Autodesk Inventor part; units mm, degrees
ref_plane "YZ Plane" through (0, 0, 0) normal (1, 0, 0) x (0, 1, 0)
ref_plane "XZ Plane" through (0, 0, 0) normal (0, 1, 0) x (-1, 0, 0)
ref_plane "XY Plane" through (0, 0, 0) normal (0, 0, 1) x (1, 0, 0)
sketch "Эскиз1" plane through (0, 0, 0) normal (0, 0, 1) x (1, 0, 0)
  circle A0 centre (-3.8814, -5.2176) radius 1.5
  line L0 (-10.8201, 1.8432) -> (-11.0949, -29.6556)
  line L1 (4.4719, -79.3628) -> (5.5191, 40.6326)
  line L2 (-9.8587, -12.7657) -> (-5.4656, -12.804)
  line L3 (-10.9475, -12.7562) -> (5.315, -12.7562)
  line L4 (5.315, -12.7562) -> (5.315, 17.2438)
  line L5 (5.315, 17.2438) -> (-10.9475, 17.2438)
  line L6 (-10.9475, 17.2438) -> (-10.9475, -12.7562)
  point P0 (0, 0)
  point P1 (5.1784, 1.5986)
  point P2 (5.0531, -12.7562)
  dimension "d0" = 30
extrude "Выдавливание1" add sketch "Эскиз1" along normal blind 3 contours L3 L6 L5 L1
sketch "Эскиз2" plane through (5.315, 17.2438, 3) normal (1, -0.0087, 0) x (0, 0, -1)
  spline S0 degree 3 poles (-15.9024, -5.0587) (-16.7308, -5.0587) (-17.4024, -4.3871) (-17.4024, -3.5587) (-17.4024, -2.7303) (-16.7308, -2.0587) (-15.9024, -2.0587) (-15.074, -2.0587) (-14.4024, -2.7303) (-14.4024, -3.5587) (-14.4024, -4.3871) (-15.074, -5.0587) (-15.9024, -5.0587) knots 0 0 0 0 0.25 0.25 0.25 0.5 0.5 0.5 0.75 0.75 0.75 1 1 1 1
  spline S1 degree 3 poles (-20.7708, 4.5722) (-21.5992, 4.5722) (-22.2708, 5.2438) (-22.2708, 6.0722) (-22.2708, 6.9006) (-21.5992, 7.5722) (-20.7708, 7.5722) (-19.9424, 7.5722) (-19.2708, 6.9006) (-19.2708, 6.0722) (-19.2708, 5.2438) (-19.9424, 4.5722) (-20.7708, 4.5722) knots 0 0 0 0 0.25 0.25 0.25 0.5 0.5 0.5 0.75 0.75 0.75 1 1 1 1
  line L0 (0, -30.0011) -> (0, 0)
  line L1 (0, -7.2902) -> (-26.751, -7.2902)
  spline S2 degree 3 poles (-117.3896, -42.4533) (-114.4523, -72.8485) (-88.8364, -96.6103) (-57.6706, -96.6103) (-24.5335, -96.6103) (2.3293, -69.7475) (2.3293, -36.6104) (2.3293, -3.4733) (-24.5335, 23.3896) (-57.6706, 23.3896) (-89.3782, 23.3896) (-115.3412, -1.2057) (-117.5222, -32.3587) knots 0 0 0 0 0.2 0.2 0.2 0.4 0.4 0.4 0.6 0.6 0.6 0.8 0.8 0.8 0.8
  line L2 (-26.751, -7.2902) -> (-26.751, 14.8198)
  line L3 (-10.1308, 0) -> (0, 0)
  point P0 (3, -17.2895)
  point P1 (-15.9024, -5.0587)
  point P2 (-20.7708, 4.5722)
extrude "Выдавливание2" add sketch "Эскиз2" against normal blind 3 contours L1 S2 L3 L0 | L1 L2 S2
sketch "Эскиз3" plane through (0, 0, 0) normal (0, 0, -1) x (-1, 0, 0)
  line L0 (-5.315, 17.2438) -> (10.9475, 17.2438)
  line L1 (10.9475, -12.7562) -> (-5.0531, -12.7562)
  line L2 (10.9475, 17.2438) -> (10.9475, -12.7562)
  line L3 (-5.315, 17.2438) -> (10.9475, 17.2438)
  line L4 (-5.0531, -12.7562) -> (-5.315, 17.2438)
  circle A0 centre (3.8814, -5.2176) radius 1.5
  point P0 (0, 0)
extrude "Выдавливание3" add sketch "Эскиз3" against normal blind 6
sketch "Эскиз4" plane through (0, 0, 0) normal (0, 0, -1) x (-1, 0, 0)
  line L0 (10.9475, -12.7562) -> (-5.0531, -12.7562)
  line L1 (10.9475, 17.2438) -> (10.9475, -12.7562)
  line L2 (-5.315, 17.2438) -> (10.9475, 17.2438)
  line L3 (-5.0531, -12.7562) -> (-5.315, 17.2438)
  circle A0 centre (3.8814, -5.2176) radius 1.5
  point P0 (0, 0)
extrude "Выдавливание4" cut sketch "Эскиз4" against normal blind 3
sketch "Эскиз5" plane through (-10.9475, -12.7562, 3) normal (0, -1, 0) x (1, 0, 0)
  line L0 (0, 0) -> (16.0006, 0)
  line L1 (16.0006, 0) -> (16.0006, 3)
  line L2 (0, 3) -> (16.0006, 3)
  line L3 (0, 0) -> (0, 3)
  point P0 (10.9475, -3)
extrude "Выдавливание5" add sketch "Эскиз5" along normal blind 5
mirror "Зеркальное отражение1" about plane through (5.2513, 9.9539, 29.751) normal (0, 0, 1) of "Выдавливание3", "Выдавливание2", "Выдавливание5"
sketch "Эскиз7" plane through (5.315, 17.2438, 13.1308) normal (1, -0.0087, 0) x (0, 0, -1)
  ellipse E0 centre (-44.6759, -33.7501) end of major axis (-85.7491, 7.3732) minor radius 55.9525 (0, 0) -> (-16.6202, 14.8198) ccw
  line L0 (0, 0) -> (0, -43.3652)
  line L1 (-16.6202, 18.912) -> (20.2447, 18.912)
  line L2 (20.2447, 18.912) -> (20.2447, -40.2119)
  line L3 (20.2447, -40.2119) -> (-16.6202, -40.2119)
  line L4 (-16.6202, -40.2119) -> (-16.6202, 18.912)
  line L5 (-46.3712, -30.1408) -> (-43.3712, -30.1408)
  line L6 (-43.3712, -30.1408) -> (-60.2207, -30.1408)
  line L7 (-60.2207, -30.1408) -> (-60.2207, 23.0222)
  line L8 (-60.2207, 23.0222) -> (-43.3712, 23.0222)
  line L9 (-43.3712, 23.0222) -> (-43.3712, -30.1408)
  point P0 (13.1308, -17.2895)
extrude "Выдавливание6" cut sketch "Эскиз7" against normal blind 30
sketch "Эскиз8" plane through (5.0531, -17.7562, 6) normal (1, 0, 0) x (0, 0, -1)
  line L0 (3, 5) -> (0, 5)
  line L1 (0, 5) -> (0, 0)
  line L2 (3, 0) -> (0, 0)
  line L3 (3, 5) -> (3, 0)
  point P0 (6, 17.7562)
extrude "Выдавливание7" cut sketch "Эскиз8" against normal blind 30
properties part number "encoderholderL"
Can you work these out from the model? Positions are in its coordinate system, mm. A direction names the side the tool comes from. Give positions to 0.01 mm unless a question says otherwise; leave off trailing zeros. Order: outer loops, then holes, each group sorted by start corner. A loop starts at its lowest first (then second) coordinate and runs counter-clockwise, first axis right, second up. Notation, with made-up numbers: M 5.5,28.5 L 64.5,28.5 A16 cw 64.5,35.5 Z; hole C 28,39.5 d7. An arc over 180 degrees is marked long. Use a Markdown table: item, result. Add a question column.
Item 1: For faces 4 (the flat face through (5.053, -15, 55)), 5 (the flat face through (4, 21, 29.751)), which set-ups out of +Z, -Z, +X, -X, +Y, -Y let a thin tool reach every point of the face, with its end or its side?
Item 2: Suppose I cut it at B-B (x = -3.5). List the corners of the cut face in (y, z) for me.
Item 3: Suppose I cut it at C-C (x = -9.5). List the corners of the cut face in (y, z) for me, then the cut area to 3 significant figures.
Item 4: Will these pins go through, and if not, where does the flat tip stop? pin 1 (5.5 mm diameter, centred on x = -6, y = -15.5, fed in from -Z); pin 2 (4 mm diameter, centred on y = 10, z = 35, fed in from +X); pin 3 (1.5 mm diameter, centred on y = -14.5, z = 55.5, fed in from +X).
Item 5: We'd pull the mould along Y, two halves only. Please class faces 1 (the cylindrical face through (-2.776, -6.231, 55.023)), 2 (the flat face through (-3, -17.756, 55)), 3 (the flat face through (-4, 17.244, 55)): +Y half, -Y half, draft (parallel to the pull), parting line (faces both ways), or undercut.
Item 6: If I drill on L1, parallel to Z at x = 1, y = 5; L2, parallel to Y at x = 2.25, z = 54; L3, parallel to Z at x = 4.75, y = 23, over which ranges is the centre line in solid material (lowest first)? Write a range as [from, to].
Item 7: Suppose I cut it at D-D (y = -14). List the corners of the cut face in (x, z) for me, then the cut area to 3 significant figures.
Answer sheet:
| question | item | result |
|---|---|---|
| 1 | face 4 | +Z, -Z, +X, -Y |
| 1 | face 5 | -Z, +X, -X, +Y, -Y |
| 2 | outline | M -17.76,53.5 L -6.67,53.5 L -6.67,56.5 L -17.76,56.5 Z; M -3.77,53.5 L 17.24,53.5 L 17.24,56.5 L -3.77,56.5 Z |
| 3 | outline | M -17.76,53.5 L 17.24,53.5 L 17.24,56.5 L -17.76,56.5 Z |
| 3 | area | 105 mm² |
| 4 | pin 1 | stops at z = 53.5 |
| 4 | pin 2 | stops at x = 5.27 |
| 4 | pin 3 | stops at x = 5.05 |
| 5 | face 1 | undercut |
| 5 | face 2 | -Y half |
| 5 | face 3 | +Y half |
| 6 | L1 | z = [53.5, 56.5] |
| 6 | L2 | y = [-17.76, 17.24] |
| 6 | L3 | z = [29.75, 34.27], [37.2, 41.32] |
| 7 | outline | M -10.95,53.5 L 5.05,53.5 L 5.05,56.5 L -10.95,56.5 Z |
| 7 | area | 48.0 mm² |
